from build123d import *

# Parameters (mm, degrees)
F0_W     = 100
F0_H     = 100
F1_DEPTH = 100
F2_W     = 98
F2_H     = 98
F3_DEPTH = 98


with BuildPart() as f1:
    # F0 (on Front) → F1 (new body)
    with BuildSketch(Plane.XZ):
        Rectangle(F0_W, F0_H)
    extrude(amount=-F1_DEPTH)

    # F2 (on face) → F3 (cut)
    with BuildSketch(Plane.XY.offset(50)):
        with Locations((0, 50)):
            Rectangle(F2_W, F2_H)
    extrude(amount=-F3_DEPTH, mode=Mode.SUBTRACT)


solid = f1.part
Read the model definition and answer for the solid it produces. Units are mm, in the model's axes. A direction names the side the tool comes from. Give positions to 0.01 mm unless a question says otherwise; leave off trailing zeros. Write each loop counter-clockwise with the first axis right and the second up, starting at its lowest first coordinate (ties: lowest second). Pieces come first, ordered by that corner, then holes. Notation, with made-up numbers: M -24,51 L 0,51 A19 cw 0,56 Z; hole C 27.25,3 d3. An arc over 180 degrees is marked long. One line per item, written item: value. Start each with the question number.
(1) Find the intervals of material crossed by line 1 (Y direction, x = 43, z = -26.5); line 2 (X direction, y = 60.5, z = -23); line 3 (Z direction, x = 14, y = 84), in increasing order.
(2) Determine the mould class of faces 1 (the flat face through (-1, 1, 2)), 2 (the flat face through (-50, 49, -1)), 3 (the flat face through (-1, 0, 1)) for opening direction X: pulls with the +X half, pulls with the -X half, needs draft (parallel to the pull), parting line crosses it, or undercut.
(3) Find section B-B (x = 38). Determine the outline of the cut face in (y, z), plus the area to 3 significant figures.
(4) Find section C-C (y = 39). Determine the outline of the cut face in (x, z).
(5) A tool of negligible diameter and unlimited length cuts with its end or side. For faces 4 (the flat face through (-1, 100, 1)), 5 (the flat face through (49, 49, 2)), from which of +Z, -Z, +X, -X, +Y, -Y can it reach the whole face along a straight path? Write none if from no direction.
(6) Find section A-A (z = 42). Determine the outline of the cut face in (x, y), plus the area to 3 significant figures.
(7) A flat-ended cylindrical pin translates along its axis: pin 1 Ø2 at (x, y) = (40, 30) entering from +Z. Find the tip coordinate at first contact, or state that the pin passes through.
Results below:
1. line 1: y = 0 to 1, 99 to 100
1. line 2: x = -50 to -49, 49 to 50
1. line 3: z = -50 to -48
2. face 1: undercut
2. face 2: pulls with the -X half
2. face 3: needs draft
3. outline: M 0,-50 L 100,-50 L 100,50 L 99,50 L 99,-48 L 1,-48 L 1,50 L 0,50 Z
3. area: 396 mm^2
4. outline: M -50,-50 L 50,-50 L 50,50 L 49,50 L 49,-48 L -49,-48 L -49,50 L -50,50 Z
5. face 4: +Z, -Z, +X, -X, +Y
5. face 5: +Z
6. outline: M -50,0 L 50,0 L 50,100 L -50,100 Z; hole M -49,1 L 49,1 L 49,99 L -49,99 Z
6. area: 396 mm^2
7. pin 1: stops at z = -48
